Autodesk Inventor part; units mm, degrees
sketch "スケッチ1" plane through (0, 0, 0) normal (0, 0, 1) x (1, 0, 0)
  line L0 (-2, 5.1) -> (2, 5.1)
  line L1 (2, 5.1) -> (2, -5.1)
  line L2 (2, -5.1) -> (-2, -5.1)
  line L3 (-2, -5.1) -> (-2, 5.1)
  point P0 (0, 0)
  dimension "d0" = 2
  dimension "d1" = 4
  dimension "d2" = 5.1
  dimension "d3" = 10.2
extrude "押し出し1" add sketch "スケッチ1" along normal blind 4.5
sketch "スケッチ4" plane through (0, 0, 0) normal (0, 0, 1) x (1, 0, 0)
  circle A0 centre (0, 2.54) radius 0.3
  circle A1 centre (0, 0) radius 0.3
  circle A2 centre (0, -2.54) radius 0.3
  dimension "d16" = 0.6
  dimension "d17" = 0.6
  dimension "d18" = 0.6
  dimension "d19" = 2.54
  dimension "d20" = 2.54
extrude "押し出し3" add sketch "スケッチ4" against normal blind 3
sketch "スケッチ5" plane through (0, 0, 0) normal (0, 0, 1) x (1, 0, 0)
  line L0 (-0.6, 1.75) -> (0.6, 1.75)
  line L1 (0.6, 1.75) -> (0.6, 0.25)
  line L2 (0.6, 0.25) -> (-0.6, 0.25)
  line L3 (-0.6, 0.25) -> (-0.6, 1.75)
  line L4 (0.6, 0.25) -> (-0.6, 1.75)
  line L5 (0.6, 1.75) -> (-0.6, 0.25)
  line L6 (0, -0.35) -> (0, 2.1)
  line L7 (-0.84, 0) -> (0.84, 0)
  point P0 (0, 0)
  point P1 (0, 1)
  point P2 (0, 1)
  dimension "d23" = 1
  dimension "d24" = 1.5
  dimension "d25" = 1.2
extrude "押し出し4" add sketch "スケッチ5" along normal blind 6.5
properties part number "SS-12SDP2"
Verification items for the finished model (mm, model axes). A direction names the side the tool comes from. Round coordinates to 2 decimals unless told otherwise and drop trailing zeros. Loops run counter-clockwise (first coordinate to the right, second up) from the corner with the lowest first, then second, coordinate; pieces in that order, holes last. Notation, with made-up numbers: (16, -40) -> (40, -40) arc R15 cw to (40, -33) -> close; hole circle Ø8 at (77.25, -23). An arc over 180 degrees is marked (long way). Answer as a JSON object with one key per item and string values.
Q1. Go/stop test with flat-tipped pins: P1, Ø1.6, axis at y = 1.5, z = 6, coming from the -X side; P2, Ø0.6, axis at x = 0, z = 5.5, coming from the -Y side; P3, Ø0.6, axis at x = 0, z = 6, coming from the +Y side. Record where each tip stops, or that it passes through.
Data:
{"P1": "stops at x = -0.6", "P2": "stops at y = 0.25", "P3": "stops at y = 1.75"}
Q2. Section check C-C (z = -0.5). Record the boundary of the cut face in (x, y).
Data:
{"outline": "circle Ø0.6 at (0, -2.54); circle Ø0.6 at (0, 0); circle Ø0.6 at (0, 2.54)"}
Q3. Section check D-D (z = 5). Record the boundary of the cut face in (x, y).
Data:
{"outline": "(-0.6, 0.25) -> (0.6, 0.25) -> (0.6, 1.75) -> (-0.6, 1.75) -> close"}
Q4. Access from +Z, -Z, +X, -X, +Y, -Y to the whole of each face (thin tool, end or side, straight path). Record for faces 1 (the flat face through (-0.6, 1, 5)), 2 (the flat face through (0, 1.75, 5)), 3 (the flat face through (2, 0, 2)), 4 (the flat face through (0, 0.25, 5)), 5 (the flat face through (0.6, 1, 5)).
Data:
{"face 1": "+Z, -X, +Y, -Y", "face 2": "+Z, +X, -X, +Y", "face 3": "+Z, -Z, +X, +Y, -Y", "face 4": "+Z, +X, -X, -Y", "face 5": "+Z, +X, +Y, -Y"}
Q5. Scan lines: line 1 (Z direction, x = 0.8, y = -0.5); line 2 (Y direction, x = 0.1, z = -2.25); line 3 (Z direction, x = 0.1, y = 2.75). Record each from-to range of solid material in increasing order. Write a range as from..to.
Data:
{"line 1": "z = 0..4.5", "line 2": "y = -2.82..-2.26, -0.28..0.28, 2.26..2.82", "line 3": "z = -3..4.5"}
Q6. Section check B-B (y = 2.54). Record the boundary of the cut face in (x, z), then the cut area to 3 significant figures.
Data:
{"outline": "(-2, 0) -> (-0.3, 0) -> (-0.3, -3) -> (0.3, -3) -> (0.3, 0) -> (2, 0) -> (2, 4.5) -> (-2, 4.5) -> close", "area": "19.8 mm2"}
Q7. Section check A-A (x = 0). Record the boundary of the cut face in (y, z).
Data:
{"outline": "(-5.1, 0) -> (-2.84, 0) -> (-2.84, -3) -> (-2.24, -3) -> (-2.24, 0) -> (-0.3, 0) -> (-0.3, -3) -> (0.3, -3) -> (0.3, 0) -> (2.24, 0) -> (2.24, -3) -> (2.84, -3) -> (2.84, 0) -> (5.1, 0) -> (5.1, 4.5) -> (1.75, 4.5) -> (1.75, 6.5) -> (0.25, 6.5) -> (0.25, 4.5) -> (-5.1, 4.5) -> close"}
